```python
from build123d import *

# Parameters (mm, degrees)
SKETCH2_R           = 25
BOSS_EXTRUDE1_DEPTH = 4
SKETCH4_R           = 25
BOSS_EXTRUDE2_DEPTH = 6
BOSS_EXTRUDE2_TAPER = 69
SKETCH5_R           = 9.369465612
BOSS_EXTRUDE3_DEPTH = 2
SKETCH6_R           = 5
BOSS_EXTRUDE4_DEPTH = 44
FILLET1_R           = 2
BOSS_EXTRUDE5_DEPTH = 5


with BuildPart() as part:
    # Sketch2 → Boss-Extrude1 (new body)
    with BuildSketch(Plane(origin=(0, 0, 0), x_dir=(1, 0, 0), z_dir=(0, 1, 0))):
        with Locations(Location((0, 0, 0), (0, 0, 270))):
            Circle(SKETCH2_R)
    extrude(amount=BOSS_EXTRUDE1_DEPTH)

    # Sketch4 → Boss-Extrude2 (add)
    with BuildSketch(Plane(origin=(0, 4, 0), x_dir=(1, 0, 0), z_dir=(0, 1, 0))):
        with Locations(Location((0, 0, 0), (0, 0, 270))):
            Circle(SKETCH4_R)
    extrude(amount=BOSS_EXTRUDE2_DEPTH, taper=BOSS_EXTRUDE2_TAPER)

    # Sketch5 → Boss-Extrude3 (add)
    with BuildSketch(Plane(origin=(0, 10, 0), x_dir=(1, 0, 0), z_dir=(0, 1, 0))):
        with Locations(Location((0, 0, 0), (0, 0, 270))):
            Circle(SKETCH5_R)
    extrude(amount=BOSS_EXTRUDE3_DEPTH)

    # Sketch6 → Boss-Extrude4 (add)
    with BuildSketch(Plane(origin=(0, 12, 0), x_dir=(1, 0, 0), z_dir=(0, 1, 0))):
        with Locations(Location((0, 0, 0), (0, 0, 270))):
            Circle(SKETCH6_R)
    extrude(amount=BOSS_EXTRUDE4_DEPTH)

    # Fillet1
    fillet1_edges = [part.edges().sort_by_distance(p)[0] for p in [
        (0, 12, -9.369465612),
    ]]
    fillet(fillet1_edges, radius=FILLET1_R - 0.0001)  # a hair under: the kernel refuses the full size

    # Sketch7 → Boss-Extrude5 (add)
    with BuildSketch(Plane(origin=(0, 12, 0), x_dir=(1, 0, 0), z_dir=(0, 1, 0))):
        Polygon((6.645053271, 0), (3.322526636, 5.754784943), (-3.322526636, 5.754784943), (-6.645053271, 0), (-3.322526636, -5.754784943), (3.322526636, -5.754784943), align=None)
    extrude(amount=BOSS_EXTRUDE5_DEPTH)


solid = part.part
```
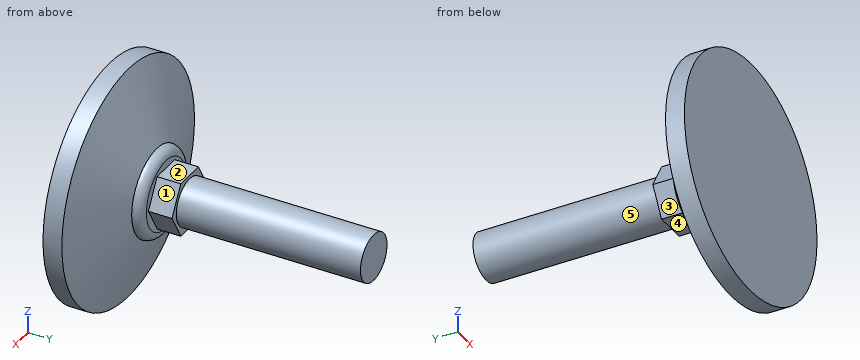
Part model, mm, in its own coordinate system. Face numbers are marked on the shaded views. A direction names the side the tool comes from. Coordinates: 2 decimals unless noted, no trailing zeros. Write each loop counter-clockwise with the first axis right and the second up, starting at its lowest first coordinate (ties: lowest second). Pieces come first, ordered by that corner, then holes.
Item 1: Slice it at A-A (y = 13). Write the cut outline in (x, z).
Item 2: Pin check, flat tips, straight feed: pin 1 (2.5 mm diameter, centred on x = -1, y = 15, fed in from -Z); pin 2 (10 mm diameter, centred on x = -8, z = -8.5, fed in from +Y); pin 3 (5 mm diameter, centred on x = -7, y = 20, fed in from -Z). Stop position of each tip, or through.
Item 3: Which spindle directions (+Z, -Z, +X, -X, +Y, -Y) get a long thin tool onto all of the face, cutting with end or side? Do the marked faces 1, 2, 3, 4 and 5. Say none if no direction does.
Item 4: Slice it at B-B (y = 23). Write the cut outline in (x, z), and give its area (3 significant figures).
Item 5: Probe line 1 (Z direction, x = -2.5, y = 16); line 2 (Y direction, x = 7.5, z = 1); line 3 (X direction, y = 50.5, z = 0). List the from-to ranges inside material, lowest first.
Results found:
1. outline: (-6.65, 0) - (-3.32, -5.75) - (3.32, -5.75) - (6.65, 0) - (3.32, 5.75) - (-3.32, 5.75) - close
2. pin 1: stops at z = -5.75
2. pin 2: stops at y = 12
2. pin 3: stops at z = -2.18
3. face 1: +Z, +X, +Y
3. face 2: +Z, +X, -X, +Y
3. face 3: -Z, -X, +Y
3. face 4: -Z, +X, -X, +Y
3. face 5: +Y
4. outline: circle Ø10 at (0, 0)
4. area: 78.5 mm2
5. line 1: z = -5.75 to 5.75
5. line 2: y = 0 to 11.99
5. line 3: x = -5 to 5
